Check sheet for the modelled part. Datum: model origin and axes. Units: mm. Face numbers are marked on the shaded views. A direction names the side the tool comes from. Round coordinates to 2 decimals unless told otherwise and drop trailing zeros. Order: outer loops, then holes, each group sorted by start corner. A loop starts at its lowest first (then second) coordinate and runs counter-clockwise, first axis right, second up.
(1) Sectioned sample at A-A, the plane x = 0. Enter the section's corners in (y, z) (3 decimals).
(2) Thickness scan on probe 1 along Z at (x, y) = (0.1, 37); probe 2 along X at (y, z) = (30, 1.65); probe 3 along Y at (x, z) = (2.1, 0.2). Record the ranges inside material, lowest first.
(3) Tool access check on the marked faces 1, 2 and 3. Record the directions out of +Z, -Z, +X, -X, +Y, -Y that give a thin tool (end or side, any length) a straight path to the whole face; none if there is none.
(4) Depth check by flat-ended pin: pin 1 (1.5 mm diameter, centred on x = 2, z = 1.5, fed in from -Y); pin 2 (1.5 mm diameter, centred on x = -1.5, y = 22.5, fed in from -Z). Enter the tip coordinate at first touch or a pass-through.
(5) Sectioned sample at C-C, the plane y = 26. Enter the section's corners in (x, z).
(6) Sectioned sample at B-B, the plane z = 0. Enter the section's corners in (x, y) (3 decimals).
```python
from build123d import *

# Parameters (mm, degrees)
CROQUIS1_R              = 2.5
SALIENTE_EXTRUIR1_DEPTH = 66
CROQUIS2_R              = 1.875
SALIENTE_EXTRUIR2_DEPTH = 4
CROQUIS3_R              = 1.875
SALIENTE_EXTRUIR3_DEPTH = 4


with BuildPart() as part:
    # Croquis1 → Saliente-Extruir1 (new body)
    with BuildSketch(Plane(origin=(0, 0, 0), x_dir=(1, 0, 0), z_dir=(0, 1, 0))):
        Circle(CROQUIS1_R)
    extrude(amount=SALIENTE_EXTRUIR1_DEPTH)

    # Croquis2 → Saliente-Extruir2 (add)
    with BuildSketch(Plane(origin=(0, 66, 0), x_dir=(1, 0, 0), z_dir=(0, 1, 0))):
        Circle(CROQUIS2_R)
    extrude(amount=SALIENTE_EXTRUIR2_DEPTH)

    # Croquis3 → Saliente-Extruir3 (add)
    with BuildSketch(Plane.XZ):
        Circle(CROQUIS3_R)
    extrude(amount=SALIENTE_EXTRUIR3_DEPTH)


solid = part.part
```
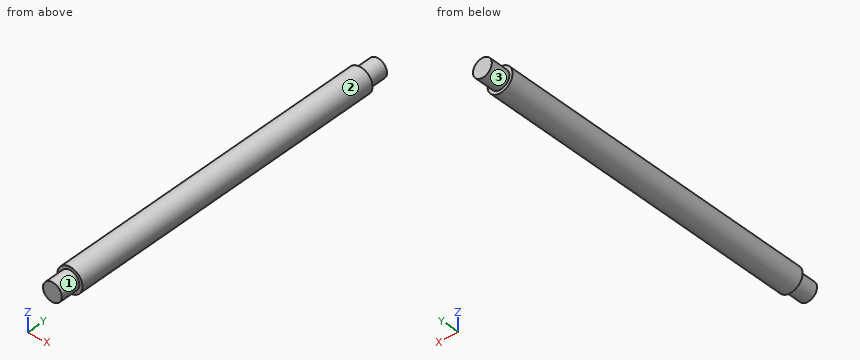
Derived:
1. outline: (-4, -1.875) - (0, -1.875) - (0, -2.5) - (66, -2.5) - (66, -1.875) - (70, -1.875) - (70, 1.875) - (66, 1.875) - (66, 2.5) - (0, 2.5) - (0, 1.875) - (-4, 1.875) - close
2. probe 1: z = -2.5 to 2.5
2. probe 2: x = -1.88 to 1.88
2. probe 3: y = 0 to 66
3. face 1: -Y
3. face 2: +Y, -Y
3. face 3: +Y
4. pin 1: stops at y = -4
4. pin 2: stops at z = -2.38
5. outline: circle Ø5 at (0, 0)
6. outline: (-2.5, 0) - (-1.875, 0) - (-1.875, -4) - (1.875, -4) - (1.875, 0) - (2.5, 0) - (2.5, 66) - (1.875, 66) - (1.875, 70) - (-1.875, 70) - (-1.875, 66) - (-2.5, 66) - close
